Autodesk Inventor part; units mm, degrees
ref_plane "YZ Plane" through (0, 0, 0) normal (1, 0, 0) x (0, 1, 0)
ref_plane "XZ Plane" through (0, 0, 0) normal (0, 1, 0) x (-1, 0, 0)
ref_plane "XY Plane" through (0, 0, 0) normal (0, 0, 1) x (1, 0, 0)
sketch "Sketch1" plane through (0, 0, 0) normal (0, 1, 0) x (-1, 0, 0)
  line L0 (0, 0) -> (-41, 0)
  line L1 (-41, 0) -> (-41, 41)
  line L2 (-41, 41) -> (0, 41)
  line L3 (0, 41) -> (0, 0)
  circle A0 centre (-20.5, 20.5) radius 17.5
  point P0 (-20.5, 0)
  dimension "d0" = 41
  dimension "d1" = 41
  dimension "d2" = 20.5
  dimension "d3" = 20.5
  dimension "d4" = 35
extrude "Extrusion1" add sketch "Sketch1" against normal blind 20
sketch "Sketch3" plane through (0, 0, 41) normal (0, 0, 1) x (1, 0, 0)
  circle A0 centre (20.5, -10) radius 4.5
  point P0 (0, 0)
  dimension "d8" = 9
extrude "Extrusion2" cut sketch "Sketch3" against normal blind 5
sketch "Sketch4" plane through (41, 0, 0) normal (0, 0, -1) x (-1, 0, 0)
  circle A0 centre (20.5, -10) radius 4.5
  circle A1 centre (20.5, -10) radius 2.5
  point P0 (41, 0)
  dimension "d11" = 5
extrude "Extrusion3" cut sketch "Sketch4" against normal blind 5 contours A1
sketch "Sketch5" plane through (0, 0, 41) normal (0, 0, 1) x (1, 0, 0)
  line L0 (41, 0) -> (0, 0)
  line L1 (0, -20) -> (41, -20)
  line L2 (0, 0) -> (41, 0)
  line L3 (41, 0) -> (41, -20)
  line L4 (41, -20) -> (0, -20)
  line L5 (0, -20) -> (0, 0)
  line L6 (0, 0) -> (0, -20)
  line L7 (0, 0) -> (41, 0)
  line L8 (41, 0) -> (41, -20)
  line L9 (41, -20) -> (0, -20)
  line L10 (0, -20) -> (0, 0)
  circle A0 centre (20.5, -10) radius 4.5
extrude "Extrusion4" add sketch "Sketch5" along normal blind 2
sketch "Sketch6" plane through (0, 0, 43) normal (0, 0, 1) x (1, 0, 0)
  line L0 (0, 0) -> (0, -20)
  line L1 (0, -20) -> (41, -20)
  line L2 (0, 0) -> (41, 0)
  line L3 (41, 0) -> (41, -20)
  line L4 (41, -20) -> (0, -20)
  line L5 (0, -20) -> (0, 0)
  circle A0 centre (20.5, -10) radius 2.5
extrude "Extrusion5" add sketch "Sketch6" along normal blind 5
equation "\"d1\" = d0"
properties part number "welco mount v01"
Verification items for the finished model (mm, model axes). Round coordinates to 2 decimals unless told otherwise and drop trailing zeros. Order: outer loops, then holes, each group sorted by start corner. A loop starts at its lowest first (then second) coordinate and runs counter-clockwise, first axis right, second up. Notation, with made-up numbers: (-31, 12) - (-25, 12) arc R31 ccw to (-25, 49) - close; hole circle Ø6 at (71.25, -36.5). An arc over 180 degrees is marked (long way). Use CSV: the item, a comma, the result in double quotes. Start each with the question number.
1) Section check B-B, the plane x = 10. Record the cut outline in (y, z), plus the area to 3 significant figures.
2) Mould release check, pull along Y, two halves, no side actions. Record for faces 1 (the flat face through (22.4, -11.9, 43)), 2 (the cylindrical face through (16, -10, 40)), 3 (the flat face through (20, -20, 40)), 4 (the flat face through (20, -5, 48)): +Y half, -Y half, draft (parallel to the pull), parting line (faces both ways), or undercut.
3) Thickness scan on L1, parallel to Y at x = 20.5, z = 2; L2, parallel to Y at x = 20.5, z = 39.9; L3, parallel to Z at x = 35, y = -11.5. Record the ranges inside material, lowest first.
4) Go/stop test with flat-tipped pins: P1, Ø3, axis at y = -11, z = 18, coming from the -X side; P2, Ø4.5, axis at x = 20.5, y = -10, coming from the -Z side. Record where each tip stops, or that it passes through.
5) Section check A-A, the plane z = 20.5. Record the cut outline in (x, y), plus the area to 3 significant figures.
6) Section check C-C, the plane y = -10. Record the cut outline in (x, z), plus the area to 3 significant figures.
7) Section check D-D, the plane x = 20.5. Record the cut outline in (y, z).
Answers:
1,outline,"(-20, 0) - (0, 0) - (0, 6.5) - (-20, 6.5) - close; (-20, 34.5) - (0, 34.5) - (0, 48) - (-20, 48) - close"
1,area,"400 mm²"
2,face 1,"undercut"
2,face 2,"undercut"
2,face 3,"-Y half"
2,face 4,"draft"
3,L1,"y = -20 to -12.5, -7.5 to 0"
3,L2,"y = -20 to -14.5, -5.5 to 0"
3,L3,"z = 0 to 10.7, 30.3 to 48"
4,P1,"stops at x = 0"
4,P2,"passes through"
5,outline,"(0, -20) - (3, -20) - (3, 0) - (0, 0) - close; (38, -20) - (41, -20) - (41, 0) - (38, 0) - close"
5,area,"120 mm²"
6,outline,"(0, 0) - (18, 0) - (18, 3.18) arc R17.5 cw to (16, 37.41) - (16, 43) - (18, 43) - (18, 48) - (0, 48) - close; (23, 0) - (41, 0) - (41, 48) - (23, 48) - (23, 43) - (25, 43) - (25, 37.41) arc R17.5 cw to (23, 3.18) - close"
6,area,"919 mm²"
7,outline,"(-20, 0) - (-12.5, 0) - (-12.5, 3) - (-20, 3) - close; (-20, 38) - (-14.5, 38) - (-14.5, 43) - (-12.5, 43) - (-12.5, 48) - (-20, 48) - close; (-7.5, 0) - (0, 0) - (0, 3) - (-7.5, 3) - close; (-7.5, 43) - (-5.5, 43) - (-5.5, 38) - (0, 38) - (0, 48) - (-7.5, 48) - close"
